```python
from build123d import *

# Parameters (mm, degrees)
CROQUIS1_R              = 1.6
CROQUIS1_R_2            = 4.05
SALIENTE_EXTRUIR1_DEPTH = 1
REDONDEO1_R             = 3


with BuildPart() as part:
    # Croquis1 → Saliente-Extruir1 (new body, symmetric)
    with BuildSketch(Plane.XY):
        Polygon((3.5, -3.5), (20, -3.5), (20, 3.5), (3.5, 3.5), (3.5, 20), (-3.5, 20), (-3.5, 3.5), (-20, 3.5), (-20, -3.5), (-3.5, -3.5), (-3.5, -20), (3.5, -20), align=None)
        with Locations((-8, 0)):
            Circle(CROQUIS1_R, mode=Mode.SUBTRACT)
        with Locations((8, 0)):
            Circle(CROQUIS1_R, mode=Mode.SUBTRACT)
        with Locations((0, 16.25)):
            Circle(CROQUIS1_R, mode=Mode.SUBTRACT)
        with Locations((0, -16.25)):
            Circle(CROQUIS1_R, mode=Mode.SUBTRACT)
        Circle(CROQUIS1_R_2, mode=Mode.SUBTRACT)
        with Locations((0, 9.5)):
            Circle(CROQUIS1_R, mode=Mode.SUBTRACT)
        with Locations((0, -9.5)):
            Circle(CROQUIS1_R, mode=Mode.SUBTRACT)
        with Locations((-16.25, 0)):
            Circle(CROQUIS1_R, mode=Mode.SUBTRACT)
        with Locations((16.25, 0)):
            Circle(CROQUIS1_R, mode=Mode.SUBTRACT)
    extrude(amount=SALIENTE_EXTRUIR1_DEPTH, both=True)

    # Redondeo1
    redondeo1_edges = [part.edges().sort_by_distance(p)[0] for p in [
        (3.5, -20, 0),
        (-3.5, -20, 0),
        (-3.5, -3.5, 0),
        (-20, -3.5, 0),
        (-20, 3.5, 0),
        (-3.5, 3.5, 0),
        (-3.5, 20, 0),
        (3.5, 20, 0),
        (3.5, 3.5, 0),
        (20, 3.5, 0),
        (20, -3.5, 0),
        (3.5, -3.5, 0),
    ]]
    fillet(redondeo1_edges, radius=REDONDEO1_R)


solid = part.part
```
Can you work these out from the model? Positions are in its coordinate system, mm. A direction names the side the tool comes from. Give positions to 0.01 mm unless a question says otherwise; leave off trailing zeros. Order: outer loops, then holes, each group sorted by start corner. A loop starts at its lowest first (then second) coordinate and runs counter-clockwise, first axis right, second up. Notation, with made-up numbers: (-34, 66.25) - (22, 66.25) arc R16 cw to (22, 81.25) - close; hole circle Ø2 at (78, -5). An arc over 180 degrees is marked (long way). Use a Markdown table: item, result. Add a question column.
Q1. If we mould it in two halves opening along X, with no side actions, what happens to faces 1 (the cylindrical face through (14.65, 0.07, -0.01)), 2 (the flat face through (-3.5, 12, 0)), 3 (the flat face through (-12, -3.5, 0)), 4 (the cylindrical face through (2.64, -19.1, -0.01))? For each: released by +X, released by -X, zero draft, split by the parting line, or undercut.
Q2. If we section it at B-B on z = 0.35: Count the separate pieces of the cut face and the enclosed holes in it, plus the area to 3 significant figures.
Q3. On a 3-axis mill with a long thin cutter (end or side, diameter ignored), from which of +Z, -Z, +X, -X, +Y, -Y can I reach the whole of each face in a straight line? I mean faces 5 (the flat face through (12, 3.5, 0)), 6 (the cylindrical face through (-0.35, -11.06, -0.01)), 7 (the flat face through (3.5, -12, 0)). Say none if no direction works.
Q4. Please list where these lines run through material, in increasing order: line 1 along Y through (x, z) = (0, 0.2); line 2 along Y through (x, z) = (8, -0.6); line 3 along Y through (x, z) = (-15.5, -0.6).
Q5. If we section it at A-A on x = 0: Write out the boundary of the cut face in (y, z), plus the area to 3 significant figures.
Q6. If we section it at C-C on y = 16.25: Write out the boundary of the cut face in (x, z), plus the area to 3 significant figures.
Q7. I'm going to push flat-ended pins straight in: pin 1 (1 mm diameter, centred on x = -14, z = 0, fed in from +Y); pin 2 (1 mm diameter, centred on y = 12.5, z = 0.5, fed in from +X); pin 3 (1 mm diameter, centred on y = 10, z = 0, fed in from -X); pin 4 (5 mm diameter, centred on x = 0, y = -9.5, fed in from +Z). Where does each tip first touch, or does it pass through?
Answers follow:
| question | item | result |
|---|---|---|
| 1 | face 1 | undercut |
| 1 | face 2 | released by -X |
| 1 | face 3 | zero draft |
| 1 | face 4 | released by +X |
| 2 | separate pieces | 1 |
| 2 | enclosed holes | 9 |
| 2 | area | 387 mm^2 |
| 3 | face 5 | +Z, -Z, +X, +Y |
| 3 | face 6 | +Z, -Z |
| 3 | face 7 | +Z, -Z, +X, -Y |
| 4 | line 1 | y = -20 to -17.85, -14.65 to -11.1, -7.9 to -4.05, 4.05 to 7.9, 11.1 to 14.65, 17.85 to 20 |
| 4 | line 2 | y = -3.5 to -1.6, 1.6 to 3.5 |
| 4 | line 3 | y = -3.5 to -1.41, 1.41 to 3.5 |
| 5 | outline | (-20, -1) - (-17.85, -1) - (-17.85, 1) - (-20, 1) - close; (-14.65, -1) - (-11.1, -1) - (-11.1, 1) - (-14.65, 1) - close; (-7.9, -1) - (-4.05, -1) - (-4.05, 1) - (-7.9, 1) - close; (4.05, -1) - (7.9, -1) - (7.9, 1) - (4.05, 1) - close; (11.1, -1) - (14.65, -1) - (14.65, 1) - (11.1, 1) - close; (17.85, -1) - (20, -1) - (20, 1) - (17.85, 1) - close |
| 5 | area | 38.2 mm^2 |
| 6 | outline | (-3.5, -1) - (-1.6, -1) - (-1.6, 1) - (-3.5, 1) - close; (1.6, -1) - (3.5, -1) - (3.5, 1) - (1.6, 1) - close |
| 6 | area | 7.60 mm^2 |
| 7 | pin 1 | stops at y = 3.5 |
| 7 | pin 2 | stops at x = 3.5 |
| 7 | pin 3 | stops at x = -3.5 |
| 7 | pin 4 | stops at z = 1 |
